from build123d import *

# Parameters (mm, degrees)
RESSALTO_EXTRUS_O1_DEPTH = 30
ESBO_O2_R                = 5
CORTE_EXTRUS_O1_DEPTH    = 30


with BuildPart() as part:
    # Esboço1 → Ressalto-extrusão1 (new body)
    with BuildSketch(Plane.XY):
        with BuildLine():
            Line((-85, -45), (85, -45))
            ThreePointArc((85, -45), (88.535533906, -43.535533906), (90, -40))
            Line((90, -40), (90, 40))
            ThreePointArc((90, 40), (88.535533906, 43.535533906), (85, 45))
            Line((85, 45), (-85, 45))
            ThreePointArc((-85, 45), (-88.535533906, 43.535533906), (-90, 40))
            Line((-90, 40), (-90, -40))
            ThreePointArc((-90, -40), (-88.535533906, -43.535533906), (-85, -45))
        make_face()
    extrude(amount=RESSALTO_EXTRUS_O1_DEPTH)

    # Esboço2 → Corte-extrusão1 (cut)
    with BuildSketch(Plane.XY.offset(30)):
        with Locations((0, 30)):
            Circle(ESBO_O2_R)
        with Locations((25.980762114, 15)):
            Circle(ESBO_O2_R)
        with Locations((25.980762114, -15)):
            Circle(ESBO_O2_R)
        with Locations((0, -30)):
            Circle(ESBO_O2_R)
        with Locations((-25.980762114, -15)):
            Circle(ESBO_O2_R)
        with Locations((-25.980762114, 15)):
            Circle(ESBO_O2_R)
    extrude(amount=-CORTE_EXTRUS_O1_DEPTH, mode=Mode.SUBTRACT)


solid = part.part
Build history of the part. All positions in model axes, mm. Give positions to 0.01 mm unless a question says otherwise; leave off trailing zeros. Order: outer loops, then holes, each group sorted by start corner. A loop starts at its lowest first (then second) coordinate and runs counter-clockwise, first axis right, second up. Notation, with made-up numbers: M -31,36 L -19,36 A34 cw -19,73 Z; hole C -22.5,-15.5 d11. An arc over 180 degrees is marked long. Put each result on its own line as item: value.
Item 1: Slice it at D-D, the plane z = 12.5. Write the cut outline in (x, y), plus the area to 3 significant figures.
From the geometry:
outline: M -90,-40 A5 ccw -85,-45 L 85,-45 A5 ccw 90,-40 L 90,40 A5 ccw 85,45 L -85,45 A5 ccw -90,40 Z; hole C -25.98,-15 d10; hole C -25.98,15 d10; hole C 0,-30 d10; hole C 0,30 d10; hole C 25.98,-15 d10; hole C 25.98,15 d10
area: 15,700 mm2
Item 2: Slice it at A-A, the plane y = 30. Write the cut outline in (x, z), plus the area to 3 significant figures.
From the geometry:
outline: M -90,0 L -5,0 L -5,30 L -90,30 Z; M 5,0 L 90,0 L 90,30 L 5,30 Z
area: 5,100 mm2
Item 3: Two-plate mould, pull along X, no slides. Class faces 1 (the flat face through (90, -1, 15)), 2 (the flat face through (1, 45, 15)), 3 (the cylindrical face through (-89, -43, 15)), 4 (the cylindrical face through (-1.08, 25.12, 15.21)): +X half, -X half, draft (parallel to the pull), parting line (faces both ways), or undercut.
From the geometry:
face 1: +X half
face 2: draft
face 3: -X half
face 4: undercut
Item 4: Slice it at B-B, the plane x = 0. Write the cut outline in (y, z).
From the geometry:
outline: M -45,0 L -35,0 L -35,30 L -45,30 Z; M -25,0 L 25,0 L 25,30 L -25,30 Z; M 35,0 L 45,0 L 45,30 L 35,30 Z
Item 5: Probe line 1 (Y direction, x = 0, z = 15.75); line 2 (X direction, y = -30.5, z = 11.5); line 3 (Y direction, x = 28.5, z = 14.5). List the from-to ranges inside material, lowest first. Write a range as [from, to].
From the geometry:
line 1: y = [-45, -35], [-25, 25], [35, 45]
line 2: x = [-90, -4.97], [4.97, 90]
line 3: y = [-45, -19.32], [-10.68, 10.68], [19.32, 45]
Item 6: Slice it at C-C, the plane y = -15. Write the cut outline in (x, z).
From the geometry:
outline: M -90,0 L -30.98,0 L -30.98,30 L -90,30 Z; M -20.98,0 L 20.98,0 L 20.98,30 L -20.98,30 Z; M 30.98,0 L 90,0 L 90,30 L 30.98,30 Z
